CAD build for the part. Positions are in the model's coordinates, mm. A direction names the side the tool comes from. Round coordinates to 2 decimals unless told otherwise and drop trailing zeros. Loops run counter-clockwise (first coordinate to the right, second up) from the corner with the lowest first, then second, coordinate; pieces in that order, holes last. Notation, with made-up numbers: M -33,-33 L -10,-33 A7 ccw -10,-24 Z; hole C 66,18 d6. An arc over 180 degrees is marked long. Put each result on its own line as item: value. Start each with the question number.
Autodesk Inventor part; units mm, degrees
ref_plane "YZ Plane" through (0, 0, 0) normal (1, 0, 0) x (0, 1, 0)
ref_plane "XZ Plane" through (0, 0, 0) normal (0, 1, 0) x (-1, 0, 0)
ref_plane "XY Plane" through (0, 0, 0) normal (0, 0, 1) x (1, 0, 0)
sketch "スケッチ1" plane through (0, 0, 0) normal (0, 1, 0) x (-1, 0, 0)
  line L0 (0, 0) -> (86, 0)
  line L1 (86, 0) -> (86, -46)
  line L2 (86, -46) -> (0, -46)
  line L3 (0, -46) -> (0, 0)
  dimension "d0" = 86
  dimension "d1" = 46
extrude "押し出し1" add sketch "スケッチ1" along normal blind 30
sketch "スケッチ2" plane through (0, 30, 0) normal (0, 1, 0) x (1, 0, 0)
  line L0 (-83, 3) -> (-3, 3)
  line L1 (-3, 3) -> (-3, 43)
  line L2 (-3, 43) -> (-83, 43)
  line L3 (-83, 43) -> (-83, 3)
  line L4 (-86, 46) -> (-86, 0)
  line L5 (-86, 0) -> (0, 0)
  point P0 (-83, 23)
  point P1 (-86, 23)
  point P2 (-43, 3)
  point P3 (-43, 0)
  dimension "d4" = 80
  dimension "d5" = 40
extrude "押し出し2" cut sketch "スケッチ2" against normal blind 28
sketch "スケッチ3" plane through (0, 0, 0) normal (1, 0, 0) x (0, 0, -1)
  line L0 (46, 30) -> (0, 30)
  line L1 (0, 30) -> (0, 0)
  line L2 (0, 0) -> (46, 0)
  line L3 (46, 0) -> (46, 30)
extrude "押し出し3" add sketch "スケッチ3" along normal blind 5
sketch "スケッチ4" plane through (5, 0, 0) normal (1, 0, 0) x (0, 0, -1)
  point P0 (0, 0)
(1) Tool access for faces 1 (the flat face through (-41, 0, -23)), 2 (the flat face through (-44, 2, -23)): list every direction of +Z, -Z, +X, -X, +Y, -Y with a clear straight run to the whole face (end or side of a thin tool).
(2) Flat gauge pin, fed straight in: pin 1 Ø5 at (x, z) = (-73, -8.5) entering from +Y. Where does the tip first touch, or does it go through?
(3) Cut at B-B on x = -46.5. List the corners of the cut face in (y, z), and give its area (3 significant figures).
(4) Cut at C-C on z = -29.5. List the corners of the cut face in (x, y), and give its area (3 significant figures).
(5) Mould opens along X. For faces 3 (the flat face through (-83, 16, -23)), 4 (the flat face through (-86, 15, -23)), 5 (the flat face through (-41, 15, 0)), 6 (the flat face through (5, 15, -23)) say: +X half, -X half, draft (parallel to the pull), parting line (faces both ways), or undercut.
(6) Cut at A-A on y = 7.5. List the corners of the cut face in (x, z), and give its area (3 significant figures).
(7) Drill centre lines: line 1 along X through (y, z) = (16.5, -16.5); line 2 along Z through (x, y) = (-67, 23); line 3 along Y through (x, z) = (-61, -5.5). Where is each one in solid material? Low to high.
Taken from the geometry:
1. face 1: +Z, -Z, +X, -X, -Y
1. face 2: +Y
2. pin 1: y = 2
3. outline: M 0,-46 L 30,-46 L 30,-43 L 2,-43 L 2,-3 L 30,-3 L 30,0 L 0,0 Z
3. area: 260 mm2
4. outline: M -86,0 L 5,0 L 5,30 L -3,30 L -3,2 L -83,2 L -83,30 L -86,30 Z
4. area: 490 mm2
5. face 3: undercut
5. face 4: -X half
5. face 5: draft
5. face 6: +X half
6. outline: M -86,-46 L 5,-46 L 5,0 L -86,0 Z; hole M -83,-43 L -3,-43 L -3,-3 L -83,-3 Z
6. area: 986 mm2
7. line 1: -86 to -83, -3 to 5
7. line 2: -46 to -43, -3 to 0
7. line 3: 0 to 2
